from build123d import *

# Parameters (mm, degrees)
ESQUISSE1_W             = 10
ESQUISSE1_H             = 5
BOSS_EXTRU_1_DEPTH      = 8
ESQUISSE2_W             = 6.6
ESQUISSE2_H             = 0.8
ENL_V_MAT_EXTRU_1_DEPTH = 8
ENL_V_MAT_EXTRU_2_DEPTH = 6.5
ESQUISSE5_W             = 6
ESQUISSE5_H             = 0.5
ENL_V_MAT_EXTRU_3_DEPTH = 1
ESQUISSE6_W             = 5.6
ESQUISSE6_H             = 0.5
ENL_V_MAT_EXTRU_4_DEPTH = 3
ESQUISSE7_W             = 0.8
ESQUISSE7_H             = 1
ENL_V_MAT_EXTRU_5_DEPTH = 10
ESQUISSE8_W             = 6.8
ESQUISSE8_H             = 4.2
ENL_V_MAT_EXTRU_6_DEPTH = 1
BOSS_EXTRU_2_DEPTH      = 6.8
BOSS_EXTRU_3_DEPTH      = 2
BOSS_EXTRU_3_DEPTH_BACK = 2
ESQUISSE12_W            = 0.5
ESQUISSE12_H            = 4.2
BOSS_EXTRU_4_DEPTH      = 1
CHANFREIN1_SIZE         = 0.15
BOSS_EXTRU_5_DEPTH      = 0.5
BOSS_EXTRU_5_DEPTH_BACK = 6.3
ESQUISSE13_W            = 0.425
ESQUISSE13_H            = 0.45
CHANFREIN2_SIZE         = 0.1
ESQUISSE14_W            = 0.425
ESQUISSE14_H            = 0.43
BOSS_EXTRU_6_DEPTH      = 5.5
CONG_1_R                = 0.1
CHANFREIN3_SIZE         = 0.1


with BuildPart() as part:
    # Esquisse1 → Boss.-Extru.1 (new body)
    with BuildSketch(Plane(origin=(0, 0, 0), x_dir=(1, 0, 0), z_dir=(0, 1, 0))):
        with Locations((5, 2.5)):
            Rectangle(ESQUISSE1_W, ESQUISSE1_H)
    extrude(amount=BOSS_EXTRU_1_DEPTH)

    # Esquisse2 → Enlèv. mat.-Extru.1 (cut)
    with BuildSketch(Plane(origin=(0, 8, 0), x_dir=(1, 0, 0), z_dir=(0, 1, 0))):
        with Locations((5, 0.4)):
            Rectangle(ESQUISSE2_W, ESQUISSE2_H)
    extrude(amount=-ENL_V_MAT_EXTRU_1_DEPTH, mode=Mode.SUBTRACT)

    # Esquisse4 → Enlèv. mat.-Extru.2 (cut)
    with BuildSketch(Plane(origin=(0, 8, 0), x_dir=(1, 0, 0), z_dir=(0, 1, 0))):
        Polygon((0.5, 0.5), (1.2, 0.5), (1.2, 1.3), (8.8, 1.3), (8.8, 0.5), (9.5, 0.5), (9.5, 4.5), (0.5, 4.5), align=None)
    extrude(amount=-ENL_V_MAT_EXTRU_2_DEPTH, mode=Mode.SUBTRACT)

    # Esquisse5 → Enlèv. mat.-Extru.3 (cut)
    with BuildSketch(Plane(origin=(0, 8, 0), x_dir=(1, 0, 0), z_dir=(0, 1, 0))):
        with Locations((5, 4.75)):
            Rectangle(ESQUISSE5_W, ESQUISSE5_H)
    extrude(amount=-ENL_V_MAT_EXTRU_3_DEPTH, mode=Mode.SUBTRACT)

    # Esquisse6 → Enlèv. mat.-Extru.4 (cut)
    with BuildSketch(Plane(origin=(0, 8, 0), x_dir=(1, 0, 0), z_dir=(0, 1, 0))):
        with Locations((5, 1.05)):
            Rectangle(ESQUISSE6_W, ESQUISSE6_H)
    extrude(amount=-ENL_V_MAT_EXTRU_4_DEPTH, mode=Mode.SUBTRACT)

    # Esquisse7 → Enlèv. mat.-Extru.5 (cut)
    with BuildSketch(Plane(origin=(10, 0, 0), x_dir=(0, 0, -1), z_dir=(1, 0, 0))):
        with Locations((0.4, 0.5)):
            Rectangle(ESQUISSE7_W, ESQUISSE7_H)
    extrude(amount=-ENL_V_MAT_EXTRU_5_DEPTH, mode=Mode.SUBTRACT)

    # Esquisse8 → Enlèv. mat.-Extru.6 (cut)
    with BuildSketch(Plane.XZ):
        with Locations((5, -2.9)):
            Rectangle(ESQUISSE8_W, ESQUISSE8_H)
    extrude(amount=-ENL_V_MAT_EXTRU_6_DEPTH, mode=Mode.SUBTRACT)

    # Esquisse9 → Boss.-Extru.2 (add)
    with BuildSketch(Plane(origin=(1.6, 0, 0), x_dir=(0, 0, -1), z_dir=(1, 0, 0))):
        Polygon((4.7, 1), (3.9, 0.2), (1.9, 0.2), (1.1, 1), align=None)
    extrude(amount=BOSS_EXTRU_2_DEPTH)

    # Esquisse11 → Boss.-Extru.3 (add, two sides: drawn at the far end of the back side and taken through both)
    with BuildSketch(Plane(origin=(5, 0, 0), x_dir=(0, 0, -1), z_dir=(1, 0, 0)).offset(-BOSS_EXTRU_3_DEPTH_BACK)):
        Polygon((0.8, 5), (0.1, 3.4), (0.8, 3.4), align=None)
    extrude(amount=BOSS_EXTRU_3_DEPTH + BOSS_EXTRU_3_DEPTH_BACK)

    # Esquisse12 → Boss.-Extru.4 (add)
    with BuildSketch(Plane(origin=(0, 1, 0), x_dir=(1, 0, 0), z_dir=(0, 1, 0))):
        with Locations((5, 2.9)):
            Rectangle(ESQUISSE12_W, ESQUISSE12_H)
        with Locations((3.175, 2.9)):
            Rectangle(ESQUISSE12_W, ESQUISSE12_H)
        with Locations((6.825, 2.9)):
            Rectangle(ESQUISSE12_W, ESQUISSE12_H)
    extrude(amount=-BOSS_EXTRU_4_DEPTH)

    # Chanfrein1
    chanfrein1_edges = [part.edges().sort_by_distance(p)[0] for p in [
        (2.2, 8, -1.05),
        (7.8, 8, -1.05),
    ]]
    chamfer(chanfrein1_edges, length=CHANFREIN1_SIZE)

    # Esquisse13 → Boss.-Extru.5 (add, two sides: drawn at the far end of the back side and taken through both)
    with BuildSketch(Plane.XZ.offset(-0.2).offset(-BOSS_EXTRU_5_DEPTH_BACK)):
        with Locations((2.2625, -2.9)):
            Rectangle(ESQUISSE13_W, ESQUISSE13_H)
        with Locations((4.0875, -2.9)):
            Rectangle(ESQUISSE13_W, ESQUISSE13_H)
        with Locations((5.9125, -2.9)):
            Rectangle(ESQUISSE13_W, ESQUISSE13_H)
        with Locations((7.7375, -2.9)):
            Rectangle(ESQUISSE13_W, ESQUISSE13_H)
    extrude(amount=BOSS_EXTRU_5_DEPTH + BOSS_EXTRU_5_DEPTH_BACK)

    # Chanfrein2
    chanfrein2_edges = [part.edges().sort_by_distance(p)[0] for p in [
        (2.05, 6.5, -2.9),
        (2.2625, 6.5, -2.675),
        (2.475, 6.5, -2.9),
        (2.2625, 6.5, -3.125),
        (4.3, 6.5, -2.9),
        (4.0875, 6.5, -3.125),
        (3.875, 6.5, -2.9),
        (4.0875, 6.5, -2.675),
        (5.7, 6.5, -2.9),
        (5.9125, 6.5, -2.675),
        (6.125, 6.5, -2.9),
        (5.9125, 6.5, -3.125),
        (7.7375, 6.5, -2.675),
        (7.95, 6.5, -2.9),
        (7.7375, 6.5, -3.125),
        (7.525, 6.5, -2.9),
    ]]
    chamfer(chanfrein2_edges, length=CHANFREIN2_SIZE)

    # Esquisse14 → Boss.-Extru.6 (add)
    with BuildSketch(Plane(origin=(0, 0, -3.125), x_dir=(-1, 0, 0), z_dir=(0, 0, -1))):
        with Locations((-7.7375, -0.085)):
            Rectangle(ESQUISSE14_W, ESQUISSE14_H)
        with Locations((-5.9125, -0.085)):
            Rectangle(ESQUISSE14_W, ESQUISSE14_H)
        with Locations((-4.0875, -0.085)):
            Rectangle(ESQUISSE14_W, ESQUISSE14_H)
        with Locations((-2.2625, -0.085)):
            Rectangle(ESQUISSE14_W, ESQUISSE14_H)
    extrude(amount=BOSS_EXTRU_6_DEPTH)

    # Congé1
    # the kernel refuses this fillet: 0.1 mm, written as the material it adds along each edge
    with BuildSketch(Plane(origin=(2.475, 0.13, -3.125), x_dir=(0, 0, -1), z_dir=(-1, 0, 0))) as cong_1_piece_1:
        with BuildLine():
            CenterArc((0.09539392, -0.1), CONG_1_R, 90, 72.542396876)
            Line((0, -0.07), (0, 0))
            Line((0, 0), (0.09539392, 0))
        make_face()
    extrude(amount=0.425)
    with BuildSketch(Plane(origin=(3.875, 0.13, -3.125), x_dir=(0, 0, -1), z_dir=(1, 0, 0)), Plane(origin=(7.525, 0.13, -3.125), x_dir=(0, 0, -1), z_dir=(1, 0, 0))) as cong_1_piece_2:
        with BuildLine():
            CenterArc((0.09539392, 0.1), CONG_1_R, 197.457603124, 72.542396876)
            Line((0, 0.07), (0, 0))
            Line((0, 0), (0.09539392, 0))
        make_face()
    extrude(amount=0.425)
    with BuildSketch(Plane(origin=(6.125, 0.13, -3.125), x_dir=(0, 1, 0), z_dir=(-1, 0, 0))) as cong_1_piece_3:
        with BuildLine():
            CenterArc((0.1, 0.09539392), CONG_1_R, 180, 72.542396876)
            Line((0, 0.09539392), (0, 0))
            Line((0, 0), (0.07, 0))
        make_face()
    extrude(amount=0.425)
    # the kernel refuses this fillet: 0.1 mm, written as the material it takes off along each edge
    with BuildSketch(Plane(origin=(1.8, -0.3, -2.675), x_dir=(0, 1, 0), z_dir=(1, 0, 0)), Plane(origin=(3.625, -0.3, -2.675), x_dir=(0, 1, 0), z_dir=(1, 0, 0))) as cong_1_2_piece_1:
        with BuildLine():
            CenterArc((CONG_1_R, -CONG_1_R), CONG_1_R, 90, 90)
            Line((0, -CONG_1_R), (0, 0))
            Line((0, 0), (CONG_1_R, 0))
        make_face()
    extrude(amount=0.925, mode=Mode.SUBTRACT)
    with BuildSketch(Plane(origin=(6.375, -0.3, -2.675), x_dir=(0, 1, 0), z_dir=(-1, 0, 0)), Plane(origin=(8.2, -0.3, -2.675), x_dir=(0, 1, 0), z_dir=(-1, 0, 0))) as cong_1_2_piece_2:
        with BuildLine():
            CenterArc((CONG_1_R, CONG_1_R), CONG_1_R, 180, 90)
            Line((0, CONG_1_R), (0, 0))
            Line((0, 0), (CONG_1_R, 0))
        make_face()
    extrude(amount=0.925, mode=Mode.SUBTRACT)

    # Chanfrein3
    chanfrein3_edges = [part.edges().sort_by_distance(p)[0] for p in [
        (7.95, -0.085, -8.625),
        (7.7375, -0.3, -8.625),
        (7.525, -0.085, -8.625),
        (7.7375, 0.13, -8.625),
        (5.7, -0.085, -8.625),
        (5.9125, 0.13, -8.625),
        (6.125, -0.085, -8.625),
        (5.9125, -0.3, -8.625),
        (4.3, -0.085, -8.625),
        (4.0875, -0.3, -8.625),
        (3.875, -0.085, -8.625),
        (4.0875, 0.13, -8.625),
        (2.05, -0.085, -8.625),
        (2.2625, 0.13, -8.625),
        (2.475, -0.085, -8.625),
        (2.2625, -0.3, -8.625),
    ]]
    chamfer(chanfrein3_edges, length=CHANFREIN3_SIZE)


solid = part.part
Design review of the part built by this model. Coordinates are the model's own, in mm. A direction names the side the tool comes from. Give positions to 0.01 mm unless a question says otherwise; leave off trailing zeros. Loops run counter-clockwise (first coordinate to the right, second up) from the corner with the lowest first, then second, coordinate; pieces in that order, holes last. Notation, with made-up numbers: (-29.75, 25) - (27.25, 25) arc R20 ccw to (27.25, 63) - close; hole circle Ø5 at (-23, 82.25). An arc over 180 degrees is marked (long way). Write item = value, one per line.
1) To check wall thickness, follow line 1 (X direction, y = 3, z = -2); line 2 (Z direction, x = 1.75, y = 5.5); line 3 (Z direction, x = 4, y = 4.75) (3 decimals). State the ranges of each line that lie inside material, in increasing order.
Result sheet:
line_1 = 0 to 0.5, 9.5 to 10
line_2 = -5 to -4.5, -1.3 to -0.8
line_3 = -5 to -4.5, -3.125 to -2.675, -1.3 to -0.691
2) Draft analysis for pull direction X (two halves, no side actions). For faces 5 (the face through (0.8, 0.5, -0.8)), 6 (the face through (4.972, 4.211, -0.455)), state which applies: +X half, -X half, draft (parallel to the pull), parting line (faces both ways), or undercut.
Result sheet:
face_5 = draft
face_6 = undercut
3) Take a section at C-C on x = 2.75. State the section outline as (y, z) points, and give its area (3 significant figures).
Result sheet:
outline = (0.2, -3.9) - (1, -4.7) - (1, -5) - (7, -5) - (7, -4.5) - (1.5, -4.5) - (1.5, -1.3) - (5, -1.3) - (5, -0.8) - (1, -0.8) - (1, -1.1) - (0.2, -1.9) - close
area = 8.84 mm2
4) Take a section at B-B on z = -5.5. State the section outline as (x, y) points (3 decimals).
Result sheet:
outline = (2.05, -0.3) - (2.475, -0.3) - (2.475, 0.13) - (2.05, 0.13) - close; (3.875, -0.3) - (4.3, -0.3) - (4.3, 0.13) - (3.875, 0.13) - close; (5.7, -0.3) - (6.125, -0.3) - (6.125, 0.13) - (5.7, 0.13) - close; (7.525, -0.3) - (7.95, -0.3) - (7.95, 0.13) - (7.525, 0.13) - close
5) Take a section at A-A on y = 1.75. Count the separate pieces of the cut face and the enclosed holes in it, and give its area (3 significant figures).
Result sheet:
separate_pieces = 5
enclosed_holes = 1
area = 15.6 mm2
6) Clearance check with flat-ended pins moving along their axes: pin 1 Ø0.5 at (x, y) = (4, 4.5) entering from +Z; pin 2 Ø4 at (x, y) = (6, 5) entering from -Z; pin 3 Ø0.5 at (x, z) = (4, -5) entering from +Y; pin 4 Ø1 at (y, z) = (3.5, -7) entering from +X. State where each tip first meets the part, or that it passes through.
Result sheet:
pin_1 = -0.47
pin_2 = -5
pin_3 = 7
pin_4 = through
7) Tool access review of faces 1 (the face through (0.5, 5, -3)), 2 (the face through (2.3, 0.6, -4.3)), 3 (the face through (9.2, 0.5, -0.8)), 4 (the face through (9, 0, -3)): name each direction out of +Z, -Z, +X, -X, +Y, -Y from which nothing blocks a thin tool from reaching the whole face with its end or side.
Result sheet:
face_1 = +Y
face_2 = -Z
face_3 = +Z, +X, -X, -Y
face_4 = +Z, -Z, +X, -Y
